Geometry: final body of the model. Coordinates: model frame, mm. Face numbers are marked on the shaded views. Give positions to 0.01 mm unless a question says otherwise; leave off trailing zeros. Order: outer loops, then holes, each group sorted by start corner. A loop starts at its lowest first (then second) coordinate and runs counter-clockwise, first axis right, second up. Notation, with made-up numbers: (-13.5, -5) -> (19.5, -5) arc R24 cw to (19.5, 7) -> close; hole circle Ø8 at (-24, 66.5). An arc over 180 degrees is marked (long way). Answer in a Markdown table with one row per item. Add a question column.
Q1. Pull-direction query (X, two-part tool) for the marked faces 1, 2, 3 and 4; classes: +X half, -X half, draft (parallel to the pull), parting line (faces both ways), or undercut.
Q2. Cut plane B-B on y = -43.5. Return the cut outline in (x, z).
Q3. Cut plane A-A on z = 7.5. Return the cut outline in (x, y), and give its area (3 significant figures).
Q4. Line query: line 1 along X through (y, z) = (-53.5, 15.5); line 2 along Z through (x, y) = (54.5, -13). Output: solid intervals per line, ascending. Write a range as from..to.
Q5. Contact query for flat-ended pins moving along their axis: P1, Ø8, axis at x = 39, y = -44.5, coming from the +Z side; P2, Ø8, axis at x = -40, z = 7.5, coming from the -Y side. Output: stop coordinate, or through.
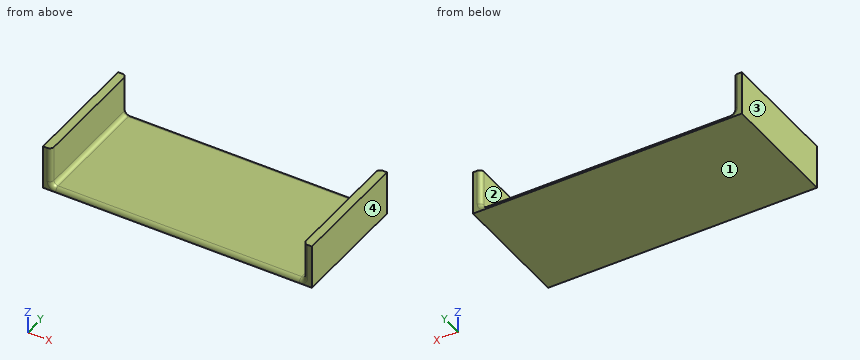
from build123d import *

# Parameters (mm, degrees)
F1_DEPTH = 58
F2_F1_R  = 2
F2_F2_R  = 1.9999


# Not quite as in the source:
# - a fillet or chamfer is up to 0.001 mm smaller than in the source, because OpenCascade refuses the exact size


with BuildPart() as f1:
    # F0 (on Front) → F1 (new body)
    with BuildSketch(Plane.XZ):
        Polygon((70.3524513997, 3.8339729243), (-49.1475486003, 3.8339729243), (-49.1475486003, 22.8339729243), (-53.1475486003, 22.8339729243), (-53.1475486003, 1.8339729243), (74.3524513997, 1.8339729243), (74.3524513997, 22.8339729243), (70.3524513997, 22.8339729243), align=None)
    extrude(amount=F1_DEPTH)

    # F2: fillet of radius 2 on 4 edges, made by hand

    # F2_f1
    f2_f1_edges = [f1.edges().sort_by_distance(p)[0] for p in [
        (70.3524513997, -29, 3.8339729243),
        (-49.1475486003, -29, 3.8339729243),
    ]]
    fillet(f2_f1_edges, radius=F2_F1_R)

    # F2_f2 (radius 2 in the source; OpenCascade refuses exactly that, so slightly less here)
    f2_f2_edges = [f1.edges().sort_by_distance(p)[0] for p in [
        (10.6024513997, 0, 3.8339729243),
        (10.6024513997, -58, 3.8339729243),
        (69.766664962, -58, 4.4197593619),
        (-48.5617621627, -58, 4.4197593619),
        (69.766664962, 0, 4.4197593619),
        (-48.5617621627, 0, 4.4197593619),
    ]]
    fillet(f2_f2_edges, radius=F2_F2_R)


solid = f1.part
Completed:
| question | item | result |
|---|---|---|
| 1 | face 1 | draft |
| 1 | face 2 | undercut |
| 1 | face 3 | -X half |
| 1 | face 4 | +X half |
| 2 | outline | (-53.15, 1.83) -> (74.35, 1.83) -> (74.35, 22.83) -> (70.35, 22.83) -> (70.35, 5.83) arc R2 cw to (68.35, 3.83) -> (-47.15, 3.83) arc R2 cw to (-49.15, 5.83) -> (-49.15, 22.83) -> (-53.15, 22.83) -> close |
| 3 | outline | (-53.15, -58) -> (-51.15, -58) arc R2 ccw to (-49.15, -56) -> (-49.15, -2) arc R2 ccw to (-51.15, 0) -> (-53.15, 0) -> close; (70.35, -56) arc R2 ccw to (72.35, -58) -> (74.35, -58) -> (74.35, 0) -> (72.35, 0) arc R2 ccw to (70.35, -2) -> close |
| 3 | area | 461 mm² |
| 4 | line 1 | x = -53.15..-49.15, 70.35..74.35 |
| 4 | line 2 | z = 1.83..3.83 |
| 5 | P1 | stops at z = 3.83 |
| 5 | P2 | stops at y = -57.11 |
